```python
from build123d import *

# Parameters (mm, degrees)
F1_DEPTH = 63.5
F2_DEPTH = 25.4
F3_DEPTH = 7.9375
F5_R     = 6.35


with BuildPart() as f1:
    # F0 (on Front) → F1 (new body, symmetric)
    with BuildSketch(Plane.XZ):
        Polygon((41.275, -9.525), (41.275, 9.525), (22.225, 9.525), (-41.275, 9.525), (-41.275, -9.525), align=None)
    extrude(amount=F1_DEPTH, both=True)

    # F0 (on Front) → F2 (join, symmetric)
    with BuildSketch(Plane.XZ):
        with BuildLine():
            ThreePointArc((57.15, 61.9252), (55.2030666201, 61.8708907791), (53.2621882973, 61.7081320209))
            add(Edge.make_bspline(
                [(53.2621882973, 61.7081320209), (54.5429566501, 61.7819276715), (55.8388527662, 61.8542223335), (57.15, 61.9252)],
                knots=[109.4465392836, 109.4465392836, 109.4465392836, 109.4465392836, 111.5045361635, 111.5045361635, 111.5045361635, 111.5045361635], degree=3))
        make_face()
        Polygon((41.275, -9.525), (41.275, 9.525), (22.225, 9.525), (-41.275, 9.525), (-41.275, -9.525), align=None)
        with BuildLine():
            Line((22.225, 9.525), (41.275, 9.525))
            Line((41.275, 9.525), (41.275, 27.0002))
            ThreePointArc((41.275, 27.0002), (45.9246798487, 38.2255201513), (57.15, 42.8752))
            Line((57.15, 42.8752), (60.325, 42.8752))
            Line((60.325, 42.8752), (60.325, 61.9252))
            Line((60.325, 61.9252), (57.15, 61.9252))
            add(Edge.make_bspline(
                [(53.2621882973, 61.7081320209), (54.5429566501, 61.7819276715), (55.8388527662, 61.8542223335), (57.15, 61.9252)],
                knots=[109.4465392836, 109.4465392836, 109.4465392836, 109.4465392836, 111.5045361635, 111.5045361635, 111.5045361635, 111.5045361635], degree=3))
            ThreePointArc((53.2621882973, 61.7081320209), (31.11600829, 50.2808121191), (22.225, 27.0002))
            Line((22.225, 27.0002), (22.225, 9.525))
        make_face()
        Polygon((60.325, 61.9252), (60.325, 42.8752), (60.325, 38.1), (85.725, 38.1), (85.6142267585, 66.675), (60.325, 66.675), align=None)
    extrude(amount=F2_DEPTH, both=True)

    # F0 (on Front) → F3 (join, symmetric)
    with BuildSketch(Plane.XZ):
        with BuildLine():
            ThreePointArc((57.15, 61.9252), (55.2030666201, 61.8708907791), (53.2621882973, 61.7081320209))
            add(Edge.make_bspline(
                [(53.2621882973, 61.7081320209), (54.5429566501, 61.7819276715), (55.8388527662, 61.8542223335), (57.15, 61.9252)],
                knots=[109.4465392836, 109.4465392836, 109.4465392836, 109.4465392836, 111.5045361635, 111.5045361635, 111.5045361635, 111.5045361635], degree=3))
        make_face()
        Polygon((41.275, -9.525), (41.275, 9.525), (22.225, 9.525), (-41.275, 9.525), (-41.275, -9.525), align=None)
        with BuildLine():
            Line((-41.275, 9.525), (22.225, 9.525))
            Line((22.225, 9.525), (22.225, 27.0002))
            ThreePointArc((22.225, 27.0002), (31.11600829, 50.2808121191), (53.2621882973, 61.7081320209))
            add(Edge.make_bspline(
                [(-41.275, 9.525), (-40.1783672468, 49.6139237835), (-14.8504824304, 57.7835980928), (53.2621882973, 61.7081320209)],
                knots=[0, 0, 0, 0, 109.4465392836, 109.4465392836, 109.4465392836, 109.4465392836], degree=3))
        make_face()
        Polygon((60.325, 61.9252), (60.325, 42.8752), (60.325, 38.1), (85.725, 38.1), (85.6142267585, 66.675), (60.325, 66.675), align=None)
        with BuildLine():
            Line((22.225, 9.525), (41.275, 9.525))
            Line((41.275, 9.525), (41.275, 27.0002))
            ThreePointArc((41.275, 27.0002), (45.9246798487, 38.2255201513), (57.15, 42.8752))
            Line((57.15, 42.8752), (60.325, 42.8752))
            Line((60.325, 42.8752), (60.325, 61.9252))
            Line((60.325, 61.9252), (57.15, 61.9252))
            add(Edge.make_bspline(
                [(53.2621882973, 61.7081320209), (54.5429566501, 61.7819276715), (55.8388527662, 61.8542223335), (57.15, 61.9252)],
                knots=[109.4465392836, 109.4465392836, 109.4465392836, 109.4465392836, 111.5045361635, 111.5045361635, 111.5045361635, 111.5045361635], degree=3))
            ThreePointArc((53.2621882973, 61.7081320209), (31.11600829, 50.2808121191), (22.225, 27.0002))
            Line((22.225, 27.0002), (22.225, 9.525))
        make_face()
    extrude(amount=F3_DEPTH, both=True)

    # F0 (on Front) → F4 (revolve)
    with BuildSketch(Plane.XZ):
        Polygon((85.6142267585, 66.675), (85.725, 38.1), (111.125, 38.1), (111.125, 66.675), align=None)
    revolve(axis=Axis((85.6696133792, 0, 52.3875), (-0.0038765498, 0, 0.9999924862)))

    # F5
    f5_edges = [f1.edges().sort_by_distance(p)[0] for p in [
        (41.275, -63.5, 0),
        (41.275, 63.5, 0),
        (-41.275, 63.5, 0),
        (-41.275, -63.5, 0),
    ]]
    fillet(f5_edges, radius=F5_R)


solid = f1.part
```
Model file for the job. Use its own axes, mm. A direction names the side the tool comes from. Coordinates: 2 decimals unless noted, no trailing zeros. Write each loop counter-clockwise with the first axis right and the second up, starting at its lowest first coordinate (ties: lowest second). Pieces come first, ordered by that corner, then holes. Notation, with made-up numbers: (-26, 66) - (-1, 66) arc R29 ccw to (-1, 102) - close; hole circle Ø5 at (19, 62.5). An arc over 180 degrees is marked (long way). One line per item, written item: value. Start each with the question number.
1. Tool access for faces 1 (the cylindrical face through (45.8, -0.4, 38.1)), 2 (the flat face through (-5, -7.938, 30)), 3 (the flat face through (22.225, 17, 18)): list every direction of +Z, -Z, +X, -X, +Y, -Y with a clear straight run to the whole face (end or side of a thin tool).
2. Slice it at B-B (y = 34). Write the cut outline in (x, z) (3 decimals).
3. Probe line 1 (Z direction, x = 103.5, y = -4.5); line 2 (X direction, y = -53, z = 4) (3 decimals); line 3 (Y direction, x = 16.5, z = 49). List the from-to ranges inside material, lowest first. Write a range as from..to.
4. Flat gauge pins, fed straight in: pin 1 (2 mm diameter, centred on y = -1, z = 45.5, fed in from -X); pin 2 (3.5 mm diameter, centred on x = 58.5, y = 9.5, fed in from +Z); pin 3 (4 mm diameter, centred on y = -14, z = 40, fed in from -X). Where does each tip first touch, or does it go through?
5. Slice it at A-A (z = -2). Write the cut outline in (x, y) (3 decimals), plus the area to 3 significant figures.
Answers below:
1. face 1: -Z, +Y, -Y
1. face 2: +Z, -X, -Y
1. face 3: +Z, -X, +Y
2. outline: (-41.275, -9.525) - (41.275, -9.525) - (41.275, 9.525) - (-41.275, 9.525) - close
3. line 1: z = 38.1..66.67
3. line 2: x = -41.275..41.275
3. line 3: y = -7.94..7.94
4. pin 1: stops at x = -26.61
4. pin 2: stops at z = 61.93
4. pin 3: stops at x = 24
5. outline: (-41.275, -57.15) arc R6.35 ccw to (-34.925, -63.5) - (34.925, -63.5) arc R6.35 ccw to (41.275, -57.15) - (41.275, 57.15) arc R6.35 ccw to (34.925, 63.5) - (-34.925, 63.5) arc R6.35 ccw to (-41.275, 57.15) - close
5. area: 10,400 mm^2
